```python
from build123d import *


with BuildPart() as part:
    # Sketch3 → Revolve1 (revolve)
    with BuildSketch(Plane.XY, mode=Mode.PRIVATE) as revolve1_sk:
        with BuildLine():
            Line((-60, 0), (60, 0))
            Line((60, 0), (60, -3))
            ThreePointArc((60, -3), (59.414213562, -4.414213562), (58, -5))
            Line((58, -5), (40, -5))
            Line((40, -5), (40, -13.60589702))
            ThreePointArc((40, -13.60589702), (38.182669225, -16.957904635), (34.382022472, -17.264058951))
            ThreePointArc((34.382022472, -17.264058951), (0, -10), (-34.382022472, -17.264058951))
            ThreePointArc((-34.382022472, -17.264058951), (-38.182669225, -16.957904635), (-40, -13.60589702))
            Line((-40, -13.60589702), (-40, -5))
            Line((-40, -5), (-58, -5))
            ThreePointArc((-58, -5), (-59.414213562, -4.414213562), (-60, -3))
            Line((-60, -3), (-60, 0))
        make_face()
    revolve(revolve1_sk.sketch.rotate(Axis((-60, 0, 0), (1, 0, 0)), 270), axis=Axis((-60, 0, 0), (1, 0, 0)))


solid = part.part
```
Model file for the job. Use its own axes, mm. A direction names the side the tool comes from. Coordinates: 2 decimals unless noted, no trailing zeros. Loops run counter-clockwise (first coordinate to the right, second up) from the corner with the lowest first, then second, coordinate; pieces in that order, holes last. Notation, with made-up numbers: (30.5, 30.25) - (79.5, 30.25) arc R16 cw to (79.5, 46.25) - close; hole circle Ø6 at (46, -19). An arc over 180 degrees is marked (long way). Answer as a JSON object with one key per item and string values. Group by question number.
(1) Tool access for faces 1 (the face through (40, 6, 0)), 2 (the face through (-60, 0, 0)), 3 (the face through (-49.13, 4.88, -1.08)): list every direction of +Z, -Z, +X, -X, +Y, -Y with a clear straight run to the whole face (end or side of a thin tool).
(2) Probe line 1 along X through (y, z) = (-8.5, 0); line 2 along X through (y, z) = (7, -15.5); line 3 along X through (y, z) = (-13, -8). List the from-to ranges inside material, lowest first.
(3) Cut at C-C (x = -41.5). Give the cut face in (y, z), then the cut area to 3 significant figures.
(4) Flat gauge pins, fed straight in: pin 1 (12 mm diameter, centred on x = -30, z = 9.5, fed in from +Y); pin 2 (5 mm diameter, centred on x = 25.5, z = 6.5, fed in from -Y); pin 3 (2 mm diameter, centred on y = 8, z = 12, fed in from +X). Where does each tip first touch, or does it go through?
(5) Cut at D-D (x = 22). Give the cut face in (y, z), then the cut area to 4 significant figures.
(6) Cut at A-A (z = 0). Give the cut face in (x, y), then the cut area to 3 significant figures.
Geometry says:
{
 "1": {"face 1": "+X", "face 2": "+Z, -Z, -X, +Y, -Y", "face 3": "-X"},
 "2": {"line 1": "x = -40 to 40", "line 2": "x = -38.1 to -33.8, 33.8 to 38.1", "line 3": "x = -39.64 to -29.45, 29.45 to 39.64"},
 "3": {"outline": "circle Ø10 at (0, 0)", "area": "78.5 mm^2"},
 "4": {"pin 1": "stops at y = 16.41", "pin 2": "stops at y = -13.7", "pin 3": "stops at x = 40"},
 "5": {"outline": "circle Ø25.79 at (0, 0)", "area": "522.5 mm^2"},
 "6": {"outline": "(-60, -3) arc R2 ccw to (-58, -5) - (-40, -5) - (-40, -13.61) arc R4 ccw to (-34.38, -17.26) arc R85 cw to (34.38, -17.26) arc R4 ccw to (40, -13.61) - (40, -5) - (58, -5) arc R2 ccw to (60, -3) - (60, 3) arc R2 ccw to (58, 5) - (40, 5) - (40, 13.61) arc R4 ccw to (34.38, 17.26) arc R85 cw to (-34.38, 17.26) arc R4 ccw to (-40, 13.61) - (-40, 5) - (-58, 5) arc R2 ccw to (-60, 3) - close", "area": "2,480 mm^2"}
}
